Can you work these out from the model? Positions are in its coordinate system, mm. Coordinates: 2 decimals unless noted, no trailing zeros. Return JSON: item names as keys, results as strings. Group by question number.
```python
from build123d import *

# Parameters (mm, degrees)
SKETCH1_W               = 355.6
SKETCH1_H               = 361.95
BOSS_EXTRUDE1_DEPTH     = 2.54
F_1_4_CLEARANCE_HOLE1_D = 6.7564
SKETCH9_W               = 6.604
SKETCH9_H               = 28.829
SKETCH9_W_2             = 6.35
SKETCH9_H_2             = 28.575
CUT_EXTRUDE1_DEPTH      = 254.714883728
MIRROR1_OUTLINE_W       = 6.477
MIRROR1_OUTLINE_H       = 28.829
MIRROR1_OUTLINE_W_2     = 6.604
MIRROR1_OUTLINE_R       = 3.3782
MIRROR1_DEPTH           = 2.54
SKETCH10_R              = 0.79375
CUT_EXTRUDE2_DEPTH      = 254.714883728


# Read off the part's stored shape, not the designer's step: Mirror1
with BuildPart() as part:
    # Sketch1 → Boss-Extrude1 (new body)
    with BuildSketch(Plane(origin=(0, 0, 0), x_dir=(1, 0, 0), z_dir=(0, 1, 0))):
        Rectangle(SKETCH1_W, SKETCH1_H)
    extrude(amount=BOSS_EXTRUDE1_DEPTH)

    # 1/4 Clearance Hole1 (through all)
    with Locations(Plane(origin=(0, 2.54, 0), x_dir=(1, 0, 0), z_dir=(0, 1, 0))):
        with Locations((-165.1, 125.4125), (-88.9, 142.875), (-88.9, 47.625), (-165.1, 52.3875), (-165.1, -20.6375), (-88.9, -47.625), (-88.9, -142.875), (-165.1, -93.6625)):
            Hole(F_1_4_CLEARANCE_HOLE1_D / 2)

    # Sketch9 → Cut-Extrude1 (cut, through all)
    # profile 1 of 8: a face of its own
    with BuildSketch(Plane(origin=(0, 0, 0), x_dir=(-1, 0, 0), z_dir=(0, -1, 0))):
        with Locations((174.625, -93.6625)):
            Rectangle(SKETCH9_W, SKETCH9_H)
        with Locations((174.625, -93.6625)):
            Rectangle(SKETCH9_W_2, SKETCH9_H_2, mode=Mode.SUBTRACT)
    # profile 2 of 8: a face of its own
    with BuildSketch(Plane(origin=(0, 0, 0), x_dir=(-1, 0, 0), z_dir=(0, -1, 0))):
        with Locations((174.625, -20.6375)):
            Rectangle(SKETCH9_W, SKETCH9_H)
        with Locations((174.625, -20.6375)):
            Rectangle(SKETCH9_W_2, SKETCH9_H_2, mode=Mode.SUBTRACT)
    # profile 3 of 8: a face of its own
    with BuildSketch(Plane(origin=(0, 0, 0), x_dir=(-1, 0, 0), z_dir=(0, -1, 0))):
        with Locations((174.625, 52.3875)):
            Rectangle(SKETCH9_W, SKETCH9_H)
        with Locations((174.625, 52.3875)):
            Rectangle(SKETCH9_W_2, SKETCH9_H_2, mode=Mode.SUBTRACT)
    # profile 4 of 8: a face of its own
    with BuildSketch(Plane(origin=(0, 0, 0), x_dir=(-1, 0, 0), z_dir=(0, -1, 0))):
        with Locations((174.625, 125.4125)):
            Rectangle(SKETCH9_W, SKETCH9_H)
        with Locations((174.625, 125.4125)):
            Rectangle(SKETCH9_W_2, SKETCH9_H_2, mode=Mode.SUBTRACT)
    # profile 5 of 8: a face of its own
    with BuildSketch(Plane(origin=(0, 0, 0), x_dir=(-1, 0, 0), z_dir=(0, -1, 0))):
        with Locations((79.375, 142.875)):
            Rectangle(SKETCH9_W, SKETCH9_H)
        with Locations((79.375, 142.875)):
            Rectangle(SKETCH9_W_2, SKETCH9_H_2, mode=Mode.SUBTRACT)
    # profile 6 of 8: a face of its own
    with BuildSketch(Plane(origin=(0, 0, 0), x_dir=(-1, 0, 0), z_dir=(0, -1, 0))):
        with Locations((79.375, 47.625)):
            Rectangle(SKETCH9_W, SKETCH9_H)
        with Locations((79.375, 47.625)):
            Rectangle(SKETCH9_W_2, SKETCH9_H_2, mode=Mode.SUBTRACT)
    # profile 7 of 8: a face of its own
    with BuildSketch(Plane(origin=(0, 0, 0), x_dir=(-1, 0, 0), z_dir=(0, -1, 0))):
        with Locations((79.375, -47.625)):
            Rectangle(SKETCH9_W, SKETCH9_H)
        with Locations((79.375, -47.625)):
            Rectangle(SKETCH9_W_2, SKETCH9_H_2, mode=Mode.SUBTRACT)
    # profile 8 of 8: a face of its own
    with BuildSketch(Plane(origin=(0, 0, 0), x_dir=(-1, 0, 0), z_dir=(0, -1, 0))):
        with Locations((79.375, -142.875)):
            Rectangle(SKETCH9_W, SKETCH9_H)
        with Locations((79.375, -142.875)):
            Rectangle(SKETCH9_W_2, SKETCH9_H_2, mode=Mode.SUBTRACT)
    extrude(amount=-CUT_EXTRUDE1_DEPTH, mode=Mode.SUBTRACT)


with BuildPart() as cut_extrude1_kept_piece:
    # of the separate pieces the step leaves, the one the design keeps (cut_extrude1_pieces_kept)
    add(part.part.solids().sort_by_distance((-177.8, 0, -180.975))[0])

    # Mirror1 outline → Mirror1 (cut)
    with BuildSketch(Plane(origin=(0, 0, 0), x_dir=(1, 0, 0), z_dir=(0, 1, 0))):
        with Locations((174.5615, 125.4125)):
            Rectangle(MIRROR1_OUTLINE_W, MIRROR1_OUTLINE_H)
        with Locations((174.5615, 52.3875)):
            Rectangle(MIRROR1_OUTLINE_W, MIRROR1_OUTLINE_H)
        with Locations((174.5615, -20.6375)):
            Rectangle(MIRROR1_OUTLINE_W, MIRROR1_OUTLINE_H)
        with Locations((174.5615, -93.6625)):
            Rectangle(MIRROR1_OUTLINE_W, MIRROR1_OUTLINE_H)
        with Locations((79.375, 142.875)):
            Rectangle(MIRROR1_OUTLINE_W_2, MIRROR1_OUTLINE_H)
        with Locations((79.375, 47.625)):
            Rectangle(MIRROR1_OUTLINE_W_2, MIRROR1_OUTLINE_H)
        with Locations((79.375, -47.625)):
            Rectangle(MIRROR1_OUTLINE_W_2, MIRROR1_OUTLINE_H)
        with Locations((79.375, -142.875)):
            Rectangle(MIRROR1_OUTLINE_W_2, MIRROR1_OUTLINE_H)
        with Locations((165.1, -93.6625)):
            Circle(MIRROR1_OUTLINE_R)
        with Locations((88.9, -142.875)):
            Circle(MIRROR1_OUTLINE_R)
        with Locations((88.9, -47.625)):
            Circle(MIRROR1_OUTLINE_R)
        with Locations((165.1, -20.6375)):
            Circle(MIRROR1_OUTLINE_R)
        with Locations((165.1, 52.3875)):
            Circle(MIRROR1_OUTLINE_R)
        with Locations((88.9, 47.625)):
            Circle(MIRROR1_OUTLINE_R)
        with Locations((88.9, 142.875)):
            Circle(MIRROR1_OUTLINE_R)
        with Locations((165.1, 125.4125)):
            Circle(MIRROR1_OUTLINE_R)
    extrude(amount=MIRROR1_DEPTH, mode=Mode.SUBTRACT)

    # Sketch10 → Cut-Extrude2 (cut, through all)
    with BuildSketch(Plane(origin=(0, 2.54, 0), x_dir=(1, 0, 0), z_dir=(0, 1, 0))):
        with Locations((-171.323, 139.03325)):
            Circle(SKETCH10_R)
        with Locations((-171.323, 111.79175)):
            Circle(SKETCH10_R)
        with Locations((-171.323, 66.00825)):
            Circle(SKETCH10_R)
        with Locations((-171.323, 38.76675)):
            Circle(SKETCH10_R)
        with Locations((-82.677, 156.49575)):
            Circle(SKETCH10_R)
        with Locations((-76.073, 156.49575)):
            Circle(SKETCH10_R)
        with Locations((-76.073, 129.25425)):
            Circle(SKETCH10_R)
        with Locations((-82.677, 129.25425)):
            Circle(SKETCH10_R)
        with Locations((-82.677, 61.24575)):
            Circle(SKETCH10_R)
        with Locations((-76.073, 61.24575)):
            Circle(SKETCH10_R)
        with Locations((-76.073, 34.00425)):
            Circle(SKETCH10_R)
        with Locations((-82.677, 34.00425)):
            Circle(SKETCH10_R)
        with Locations((-171.323, -7.01675)):
            Circle(SKETCH10_R)
        with Locations((-171.323, -34.25825)):
            Circle(SKETCH10_R)
        with Locations((-82.677, -34.00425)):
            Circle(SKETCH10_R)
        with Locations((-76.073, -34.00425)):
            Circle(SKETCH10_R)
        with Locations((-76.073, -61.24575)):
            Circle(SKETCH10_R)
        with Locations((-82.677, -61.24575)):
            Circle(SKETCH10_R)
        with Locations((-171.323, -80.04175)):
            Circle(SKETCH10_R)
        with Locations((-171.323, -107.28325)):
            Circle(SKETCH10_R)
        with Locations((-82.677, -129.25425)):
            Circle(SKETCH10_R)
        with Locations((-76.073, -129.25425)):
            Circle(SKETCH10_R)
        with Locations((-76.073, -156.49575)):
            Circle(SKETCH10_R)
        with Locations((-82.677, -156.49575)):
            Circle(SKETCH10_R)
        with Locations((82.677, -156.49575)):
            Circle(SKETCH10_R)
        with Locations((76.073, -156.49575)):
            Circle(SKETCH10_R)
        with Locations((76.073, -129.25425)):
            Circle(SKETCH10_R)
        with Locations((82.677, -129.25425)):
            Circle(SKETCH10_R)
        with Locations((171.323, -107.28325)):
            Circle(SKETCH10_R)
        with Locations((171.323, -80.04175)):
            Circle(SKETCH10_R)
        with Locations((82.677, -61.24575)):
            Circle(SKETCH10_R)
        with Locations((76.073, -61.24575)):
            Circle(SKETCH10_R)
        with Locations((76.073, -34.00425)):
            Circle(SKETCH10_R)
        with Locations((82.677, -34.00425)):
            Circle(SKETCH10_R)
        with Locations((171.323, -34.25825)):
            Circle(SKETCH10_R)
        with Locations((171.323, -7.01675)):
            Circle(SKETCH10_R)
        with Locations((82.677, 34.00425)):
            Circle(SKETCH10_R)
        with Locations((76.073, 34.00425)):
            Circle(SKETCH10_R)
        with Locations((76.073, 61.24575)):
            Circle(SKETCH10_R)
        with Locations((82.677, 61.24575)):
            Circle(SKETCH10_R)
        with Locations((82.677, 129.25425)):
            Circle(SKETCH10_R)
        with Locations((76.073, 129.25425)):
            Circle(SKETCH10_R)
        with Locations((76.073, 156.49575)):
            Circle(SKETCH10_R)
        with Locations((82.677, 156.49575)):
            Circle(SKETCH10_R)
        with Locations((171.323, 38.76675)):
            Circle(SKETCH10_R)
        with Locations((171.323, 66.00825)):
            Circle(SKETCH10_R)
        with Locations((171.323, 111.79175)):
            Circle(SKETCH10_R)
        with Locations((171.323, 139.03325)):
            Circle(SKETCH10_R)
    extrude(amount=-CUT_EXTRUDE2_DEPTH, mode=Mode.SUBTRACT)


solid = cut_extrude1_kept_piece.part
```
1) Suppose I cut it at A-A, the plane y = 0.9. Give the number of separate pieces and of enclosed holes in the cut face, then the cut area to 3 significant figures.
2) For pin 1 (6 mm diameter, centred on x = 165.1, z = -125.41, fed in from +Y), with a flat end and sliding along its axis, tell me the tip position at first contact or that it passes through.
3) If I drill on line 1 (Z direction, x = -88.9, y = 1.15) (3 decimals); line 2 (Z direction, x = 89.5, y = 1.6) (1 decimal); line 3 (X direction, y = 0.5, z = -146.5), over which ranges is the centre line in solid material (lowest first)? Write a range as from..to.
Returned:
{
 "1": {"separate pieces": "1", "enclosed holes": "24", "area": "125,000 mm²"},
 "2": {"pin 1": "passes through"},
 "3": {"line 1": "z = -180.975..-146.253, -139.497..-51.003, -44.247..44.247, 51.003..139.497, 146.253..180.975", "line 2": "z = -181..-146.2, -139.6..-50.9, -44.3..44.3, 50.9..139.6, 146.2..181", "line 3": "x = -177.8..-82.68, -76.07..76.07, 82.68..177.8"}
}
